```python
from build123d import *

# Parameters (mm, degrees)
ESQUISSE1_R             = 1.524
BOSS_EXTRU_1_DEPTH      = 2.1
ESQUISSE2_W             = 25.4
ESQUISSE2_H             = 25.4
BOSS_EXTRU_2_DEPTH      = 2.3
ESQUISSE3_W             = 164.95
ESQUISSE3_H             = 100
BOSS_EXTRU_3_DEPTH      = 3.45
ESQUISSE4_W             = 156.5
ESQUISSE4_H             = 89
ENL_V_MAT_EXTRU_1_DEPTH = 0.1
ESQUISSE5_W             = 29.8
ESQUISSE5_H             = 7.4
ENL_V_MAT_EXTRU_2_DEPTH = 2.1
CONG_1_R                = 1
ESQUISSE6_W             = 26.5
ESQUISSE6_H             = 5.4
BOSS_EXTRU_4_DEPTH      = 2
ESQUISSE7_W             = 11.59
ESQUISSE7_H             = 15
BOSS_EXTRU_5_DEPTH      = 6.16
ESQUISSE8_W             = 5.5
ESQUISSE8_H             = 7.88
BOSS_EXTRU_6_DEPTH      = 2.8
ESQUISSE9_W             = 13.84
ESQUISSE9_H             = 13.84
BOSS_EXTRU_7_DEPTH      = 1
ESQUISSE10_R            = 3.175
ESQUISSE10_R_2          = 1.524
BOSS_EXTRU_8_DEPTH      = 0.1
BOSS_EXTRU_8_DEPTH_BACK = 2.11


with BuildPart() as part:
    # Esquisse1 → Boss.-Extru.1 (new body)
    with BuildSketch(Plane.XY):
        with BuildLine():
            Line((-82.615, 53.25), (-82.615, -53.25))
            ThreePointArc((-82.615, -53.25), (-78.613, -57.252), (-74.611, -53.25))
            Line((-74.611, -53.25), (-74.611, -50.036793886))
            Line((-74.611, -50.036793886), (74.611, -50.036793886))
            Line((74.611, -50.036793886), (74.611, -53.25))
            ThreePointArc((74.611, -53.25), (78.613, -57.252), (82.615, -53.25))
            Line((82.615, -53.25), (82.615, 53.25))
            ThreePointArc((82.615, 53.25), (78.613, 57.252), (74.611, 53.25))
            Line((74.611, 53.25), (74.611, 50.036793886))
            Line((74.611, 50.036793886), (-74.611, 50.036793886))
            Line((-74.611, 50.036793886), (-74.611, 53.25))
            ThreePointArc((-74.611, 53.25), (-78.613, 57.252), (-82.615, 53.25))
        make_face()
        with Locations((-78.613, 53.25)):
            Circle(ESQUISSE1_R, mode=Mode.SUBTRACT)
        with Locations((-78.613, -53.25)):
            Circle(ESQUISSE1_R, mode=Mode.SUBTRACT)
        with Locations((78.613, -53.25)):
            Circle(ESQUISSE1_R, mode=Mode.SUBTRACT)
        with Locations((78.613, 53.25)):
            Circle(ESQUISSE1_R, mode=Mode.SUBTRACT)
    extrude(amount=BOSS_EXTRU_1_DEPTH)

    # Esquisse2 → Boss.-Extru.2 (add)
    with BuildSketch(Plane.XY.offset(2.1)):
        with Locations((-61.8, 27.3)):
            Rectangle(ESQUISSE2_W, ESQUISSE2_H)
        with Locations((-61.8, -27.3)):
            Rectangle(ESQUISSE2_W, ESQUISSE2_H)
        with Locations((61.8, 27.3)):
            Rectangle(ESQUISSE2_W, ESQUISSE2_H)
        with Locations((61.8, -27.3)):
            Rectangle(ESQUISSE2_W, ESQUISSE2_H)
    extrude(amount=BOSS_EXTRU_2_DEPTH)

    # Esquisse3 → Boss.-Extru.3 (add)
    with BuildSketch(Plane.XY.offset(4.4)):
        Rectangle(ESQUISSE3_W, ESQUISSE3_H)
    extrude(amount=BOSS_EXTRU_3_DEPTH)

    # Esquisse4 → Enlèv. mat.-Extru.1 (cut)
    with BuildSketch(Plane.XY.offset(7.85)):
        with Locations((-1.605, 2)):
            Rectangle(ESQUISSE4_W, ESQUISSE4_H)
    extrude(amount=-ENL_V_MAT_EXTRU_1_DEPTH, mode=Mode.SUBTRACT)

    # Esquisse5 → Enlèv. mat.-Extru.2 (cut)
    with BuildSketch(Plane(origin=(0, 0, 0), x_dir=(-1, 0, 0), z_dir=(0, 0, -1))):
        with Locations((38.315, -0.136793886)):
            Rectangle(ESQUISSE5_W, ESQUISSE5_H)
    extrude(amount=-ENL_V_MAT_EXTRU_2_DEPTH, mode=Mode.SUBTRACT)

    # Congé1
    cong_1_edges = [part.edges().sort_by_distance(p)[0] for p in [
        (-23.415, -3.836793886, 1.05),
        (-23.415, 3.563206114, 1.05),
        (-53.215, 3.563206114, 1.05),
        (-53.215, -3.836793886, 1.05),
    ]]
    fillet(cong_1_edges, radius=CONG_1_R)

    # Esquisse6 → Boss.-Extru.4 (add)
    with BuildSketch(Plane(origin=(0, 0, 0), x_dir=(-1, 0, 0), z_dir=(0, 0, -1))):
        with Locations((38.315, 6.363206114)):
            Rectangle(ESQUISSE6_W, ESQUISSE6_H)
    extrude(amount=BOSS_EXTRU_4_DEPTH)

    # Esquisse7 → Boss.-Extru.5 (add)
    with BuildSketch(Plane(origin=(0, 0, 0), x_dir=(-1, 0, 0), z_dir=(0, 0, -1))):
        with Locations((-79.02, 1.017206114)):
            Rectangle(ESQUISSE7_W, ESQUISSE7_H)
    extrude(amount=BOSS_EXTRU_5_DEPTH)

    # Esquisse8 → Boss.-Extru.6 (add)
    with BuildSketch(Plane(origin=(0, 0, 0), x_dir=(-1, 0, 0), z_dir=(0, 0, -1))):
        with Locations((-80.665, -20.318793886)):
            Rectangle(ESQUISSE8_W, ESQUISSE8_H)
    extrude(amount=BOSS_EXTRU_6_DEPTH)

    # Esquisse9 → Boss.-Extru.7 (add)
    with BuildSketch(Plane(origin=(0, 0, 0), x_dir=(-1, 0, 0), z_dir=(0, 0, -1))):
        with Locations((-52.695, 0.616793886)):
            Rectangle(ESQUISSE9_W, ESQUISSE9_H)
    extrude(amount=BOSS_EXTRU_7_DEPTH)

    # Esquisse10 → Boss.-Extru.8 (add, two sides)
    with BuildSketch(Plane.XY.offset(2.1)) as boss_extru_8_sk:
        with Locations((-78.613, 53.25)):
            Circle(ESQUISSE10_R)
        with Locations((-78.613, 53.25)):
            Circle(ESQUISSE10_R_2, mode=Mode.SUBTRACT)
        with Locations((-78.613, -53.25)):
            Circle(ESQUISSE10_R)
        with Locations((-78.613, -53.25)):
            Circle(ESQUISSE10_R_2, mode=Mode.SUBTRACT)
        with Locations((78.613, -53.25)):
            Circle(ESQUISSE10_R)
        with Locations((78.613, -53.25)):
            Circle(ESQUISSE10_R_2, mode=Mode.SUBTRACT)
        with Locations((78.613, 53.25)):
            Circle(ESQUISSE10_R)
        with Locations((78.613, 53.25)):
            Circle(ESQUISSE10_R_2, mode=Mode.SUBTRACT)
    extrude(amount=BOSS_EXTRU_8_DEPTH)
    extrude(boss_extru_8_sk.sketch, amount=-BOSS_EXTRU_8_DEPTH_BACK)


solid = part.part
```
Can you work these out from the model? Positions are in its coordinate system, mm. A direction names the side the tool comes from. Give positions to 0.01 mm unless a question says otherwise; leave off trailing zeros. Loops run counter-clockwise (first coordinate to the right, second up) from the corner with the lowest first, then second, coordinate; pieces in that order, holes last. Notation, with made-up numbers: M -9.75,-12.5 L 31.25,-12.5 A20 ccw 31.25,-8.5 Z; hole C 33,38 d9. An arc over 180 degrees is marked long. Use one line per item in the form item = value. Start each with the question number.
(1) On a 3-axis mill with a long thin cutter (end or side, diameter ignored), from which of +Z, -Z, +X, -X, +Y, -Y can I reach the whole of each face in a straight line? I mean faces 5 (the flat face through (82.475, -1, 6)), 6 (the flat face through (78, -55, -0.01)), 7 (the flat face through (79, 1, -6.16)). Say none if no direction works.
(2) I'm going to push flat-ended pins straight in: P1, Ø2.5, axis at x = -63, z = 3, coming from the -Y side; P2, Ø1.5, axis at y = -6, z = 3, coming from the -X side; P3, Ø5, axis at x = 78.613, y = -53.25, coming from the -Z side; P4, Ø1.4, axis at x = 79.5, z = -2, coming from the +Y side. Where does each tip first touch, or does it pass through?
(3) Thinking about a two-plate mould opening in Y: for faces 1 (the flat face through (79, 8.517, -3)), 2 (the flat face through (79, 55, -0.01)), 3 (the flat face through (79, -6.483, -3)), 4 (the flat face through (-1, -50, 6)), which applies, released by +Y, released by -Y, zero draft, split by the parting line, or undercut?
(4) I want a section at B-B, the plane y = 34. Write out the boundary of the cut face in (x, z) (3 decimals).
(5) Please list where these lines run through material, in increasing order: line 1 (Z direction, x = -20.5, y = 20.5); line 2 (Y direction, x = -71.5, z = 3.25); line 3 (X direction, y = 21.5, z = 3.5).
(6) I want a section at A-A, the plane x = -1. Write out the boundary of the cut face in (y, z), and give its area (3 significant figures).
Worked out:
q1.face_5 = +Z, +X, +Y, -Y
q1.face_6 = -Z, +X, -X, -Y
q1.face_7 = -Z, +X, -X, +Y, -Y
q2.P1 = -50.04
q2.P2 = through
q2.P3 = -0.01
q2.P4 = 8.52
q3.face_1 = released by +Y
q3.face_2 = zero draft
q3.face_3 = undercut
q3.face_4 = released by -Y
q4.outline = M -82.615,0 L 82.615,0 L 82.615,2.1 L 74.5,2.1 L 74.5,4.4 L 82.475,4.4 L 82.475,7.85 L 76.645,7.85 L 76.645,7.75 L -79.855,7.75 L -79.855,7.85 L -82.475,7.85 L -82.475,4.4 L -74.5,4.4 L -74.5,2.1 L -82.615,2.1 Z; hole M -49.1,2.1 L 49.1,2.1 L 49.1,4.4 L -49.1,4.4 Z
q5.line_1 = 0 to 2.1, 4.4 to 7.75
q5.line_2 = -40 to -14.6, 14.6 to 40
q5.line_3 = -74.5 to -49.1, 49.1 to 74.5
q6.outline = M -50.04,0 L 50.04,0 L 50.04,2.1 L -50.04,2.1 Z; M -50,4.4 L 50,4.4 L 50,7.85 L 46.5,7.85 L 46.5,7.75 L -42.5,7.75 L -42.5,7.85 L -50,7.85 Z
q6.area = 546 mm²
